Check sheet for the modelled part. Datum: model origin and axes. Units: mm. A direction names the side the tool comes from. Coordinates: 2 decimals unless noted, no trailing zeros. Loops run counter-clockwise (first coordinate to the right, second up) from the corner with the lowest first, then second, coordinate; pieces in that order, holes last. Notation, with made-up numbers: M 82,70 L 133,70 A20 cw 133,99 Z; hole C -28,74.25 d9. An arc over 180 degrees is marked long. Write each question's results on one line, items separated by ' | '. Start each with the question number.
from build123d import *

# Parameters (mm, degrees)
ESQUISSE1_W             = 25
ESQUISSE1_H             = 60
ESQUISSE1_R             = 3
ESQUISSE1_R_2           = 4.1
BASE_EXTRUSION_DEPTH    = 10
CHANFREIN1_SIZE         = 0.5
ESQUISSE2_R             = 6.6
ENL_V_MAT_EXTRU_1_DEPTH = 8.5


with BuildPart() as part:
    # Esquisse1 → Base-Extrusion (new body)
    with BuildSketch(Plane.XY):
        with Locations((12.5, 30)):
            Rectangle(ESQUISSE1_W, ESQUISSE1_H)
        with Locations((12.5, 50)):
            Circle(ESQUISSE1_R, mode=Mode.SUBTRACT)
        with Locations((12.5, 10)):
            Circle(ESQUISSE1_R, mode=Mode.SUBTRACT)
        with Locations((12.5, 30)):
            Circle(ESQUISSE1_R_2, mode=Mode.SUBTRACT)
    extrude(amount=BASE_EXTRUSION_DEPTH)

    # Chanfrein1
    chanfrein1_edges = [part.edges().sort_by_distance(p)[0] for p in [
        (0, 0, 5),
        (25, 0, 5),
        (12.5, 0, 0),
        (12.5, 0, 10),
        (25, 60, 5),
        (25, 30, 0),
        (25, 30, 10),
        (0, 60, 5),
        (12.5, 60, 0),
        (12.5, 60, 10),
        (0, 30, 0),
        (0, 30, 10),
        (9.5, 50, 10),
        (9.5, 10, 10),
    ]]
    chamfer(chanfrein1_edges, length=CHANFREIN1_SIZE)

    # Esquisse2 → Enlèv. mat.-Extru.1 (cut)
    with BuildSketch(Plane.XY.offset(10)):
        with Locations((12.5, 30)):
            Circle(ESQUISSE2_R)
    extrude(amount=-ENL_V_MAT_EXTRU_1_DEPTH, mode=Mode.SUBTRACT)


solid = part.part
Item 1: Section check B-B (y = 50). Record the cut outline in (x, z), plus the area to 3 significant figures.
Item 2: Section check C-C (x = 12.5). Record the cut outline in (y, z), plus the area to 4 significant figures.
Item 3: Section check D-D (y = 30). Record the cut outline in (x, z), plus the area to 3 significant figures.
Item 4: Tool access check on faces 1 (the face through (9, 27, 1.5)), 2 (the face through (10.1, 8.2, 4.7)). Record the directions out of +Z, -Z, +X, -X, +Y, -Y that give a thin tool (end or side, any length) a straight path to the whole face; none if there is none.
Item 5: Release check for a two-part mould opening along X. For faces 3 (the face through (25, 30, 5)), 4 (the face through (7, 30, 0)), 5 (the face through (9.246, 27.505, 0.74)), 6 (the face through (12.109, 52.974, 4.684)) record: +X half, -X half, draft (parallel to the pull), parting line (faces both ways), or undercut.
Item 6: Depth check by flat-ended pin: P1, Ø8, axis at x = 12.5, y = 10, coming from the -Z side; P2, Ø10.5, axis at x = 12.5, y = 30, coming from the +Z side. Enter the tip coordinate at first touch or a pass-through.
Item 7: Section check A-A (z = 4). Record the cut outline in (x, y), plus the area to 3 significant figures.
Item 8: Thickness scan on line 1 (Y direction, x = 12.5, z = 0.95); line 2 (Y direction, x = 12.5, z = 4); line 3 (Z direction, x = 13.25, y = 35). Record the ranges inside material, lowest first.
Computed values:
1) outline: M 0,0.5 L 0.5,0 L 9.5,0 L 9.5,9.5 L 9,10 L 0.5,10 L 0,9.5 Z; M 15.5,0 L 24.5,0 L 25,0.5 L 25,9.5 L 24.5,10 L 16,10 L 15.5,9.5 Z | area: 189 mm²
2) outline: M 0,0.5 L 0.5,0 L 7,0 L 7,9.5 L 6.5,10 L 0.5,10 L 0,9.5 Z; M 13,0 L 25.9,0 L 25.9,1.5 L 23.4,1.5 L 23.4,10 L 13.5,10 L 13,9.5 Z; M 34.1,0 L 47,0 L 47,9.5 L 46.5,10 L 36.6,10 L 36.6,1.5 L 34.1,1.5 Z; M 53,0 L 59.5,0 L 60,0.5 L 60,9.5 L 59.5,10 L 53.5,10 L 53,9.5 Z | area: 354.5 mm²
3) outline: M 0,0.5 L 0.5,0 L 8.4,0 L 8.4,1.5 L 5.9,1.5 L 5.9,10 L 0.5,10 L 0,9.5 Z; M 16.6,0 L 24.5,0 L 25,0.5 L 25,9.5 L 24.5,10 L 19.1,10 L 19.1,1.5 L 16.6,1.5 Z | area: 125 mm²
4) face 1: +Z | face 2: +Z, -Z
5) face 3: +X half | face 4: draft | face 5: undercut | face 6: undercut
6) P1: stops at z = 0 | P2: stops at z = 1.5
7) outline: M 0,0.5 L 0.5,0 L 24.5,0 L 25,0.5 L 25,59.5 L 24.5,60 L 0.5,60 L 0,59.5 Z; hole C 12.5,30 d13.2; hole C 12.5,10 d6; hole C 12.5,50 d6 | area: 1,310 mm²
8) line 1: y = 0 to 7, 13 to 25.9, 34.1 to 47, 53 to 60 | line 2: y = 0 to 7, 13 to 23.4, 36.6 to 47, 53 to 60 | line 3: z = 0 to 1.5
